from build123d import *

# Parameters (mm, degrees)
CYLINDER022_R     = 3
CYLINDER022_DEPTH = 8
TUBE001_R         = 3
TUBE001_R_2       = 1
TUBE001_DEPTH     = 6


with BuildPart() as cylinder022:
    # Cylinder022 → Cylinder022 (new body)
    with BuildSketch(Plane(origin=(28.57, 150.463, 13.35), x_dir=(0, 0, 1), z_dir=(-1, 0, 0))):
        Circle(CYLINDER022_R)
    extrude(amount=CYLINDER022_DEPTH)


with BuildPart() as fusion001:
    # Tube001 → Tube001 (new body)
    with BuildSketch(Plane(origin=(34.552, 150.466, 13.322), x_dir=(0, 1, 0), z_dir=(-1, 0, 0))):
        Circle(TUBE001_R)
        Circle(TUBE001_R_2, mode=Mode.SUBTRACT)
    extrude(amount=TUBE001_DEPTH)

    # Fusion001: union Cylinder022
    add(cylinder022.part)


with BuildPart() as fusion001_1:
    # Fusion001 placement: moved
    add(fusion001.part.moved(Location((-23.031, 0, -0.09))))


solid = fusion001_1.part
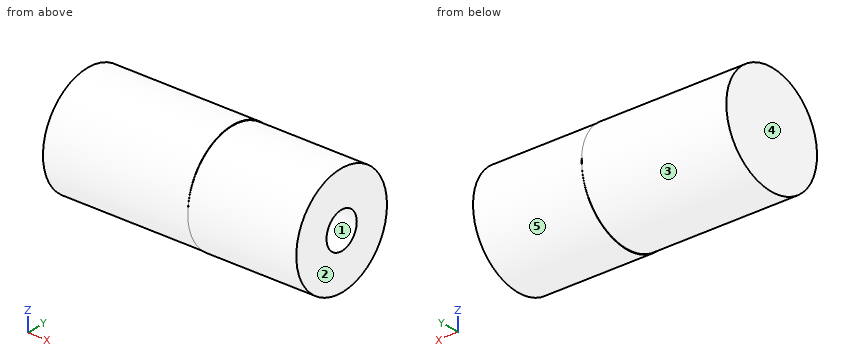
For this review, take the finished solid that the model builds, in its own axes (mm). Face numbers are marked on the shaded views. A direction names the side the tool comes from. Coordinates: 2 decimals unless noted, no trailing zeros. Loops run counter-clockwise (first coordinate to the right, second up) from the corner with the lowest first, then second, coordinate; pieces in that order, holes last. Notation, with made-up numbers: (48.5, 68.25) - (55.5, 68.25) arc R14 cw to (55.5, 84.25) - close; hole circle Ø8 at (50.25, 73). An arc over 180 degrees is marked (long way). Use a Markdown table: item, result. Add a question column.
Item 1: Mouldability with a two-part tool opening along Z and no side actions: class the marked faces 1, 2 and 3 as pulls with the +Z half, pulls with the -Z half, needs draft (parallel to the pull), parting line crosses it, or undercut.
Item 2: We need section D-D (x = -1). Give the boundary of the cut face in (y, z).
Item 3: Tool access review of the marked faces 4 and 5: name each direction out of +Z, -Z, +X, -X, +Y, -Y from which nothing blocks a thin tool from reaching the whole face with its end or side.
Item 4: We need section C-C (x = 6.75). Give the boundary of the cut face in (y, z).
Item 5: Insertion check: pin 1 Ø1 at (y, z) = (150.5, 13.5) entering from +X; pin 2 Ø1 at (x, y) = (5.5, 148) entering from +Z; pin 3 Ø1 at (x, z) = (10, 13.5) entering from -Y. Each pin has a flat end and moves straight along its axis. Give the tip position at first contact, or say it passes through.
Item 6: For line 1 (Z direction, x = 10.5, y = 149.75); line 2 (Z direction, x = 0.5, y = 150.5); line 3 (Y direction, x = 10.75, z = 12.5), list the stretches that pass through material, from the lowest coordinate up.
Results list:
| question | item | result |
|---|---|---|
| 1 | face 1 | undercut |
| 1 | face 2 | needs draft |
| 1 | face 3 | parting line crosses it |
| 2 | outline | circle Ø6 at (150.46, 13.26) |
| 3 | face 4 | +Z, -Z, -X, +Y, -Y |
| 3 | face 5 | +X |
| 4 | outline | circle Ø6 at (150.47, 13.23); hole circle Ø2 at (150.47, 13.23) |
| 5 | pin 1 | stops at x = 5.54 |
| 5 | pin 2 | stops at z = 15.53 |
| 5 | pin 3 | stops at y = 147.47 |
| 6 | line 1 | z = 10.32 to 12.53, 13.93 to 16.15 |
| 6 | line 2 | z = 10.26 to 16.26 |
| 6 | line 3 | y = 147.56 to 149.78, 151.15 to 153.38 |
